The listing builds one solid part. Answer for the finished solid, in the listing's coordinates (mm). Face numbers are marked on the shaded views. A direction names the side the tool comes from. Coordinates: 2 decimals unless noted, no trailing zeros. Order: outer loops, then holes, each group sorted by start corner. A loop starts at its lowest first (then second) coordinate and runs counter-clockwise, first axis right, second up. Notation, with made-up numbers: (-20, 73.5) -> (22, 73.5) arc R13 cw to (22, 79.5) -> close; hole circle Ø2 at (-32, 11). An arc over 180 degrees is marked (long way). Return JSON: item names as keys, results as strings.
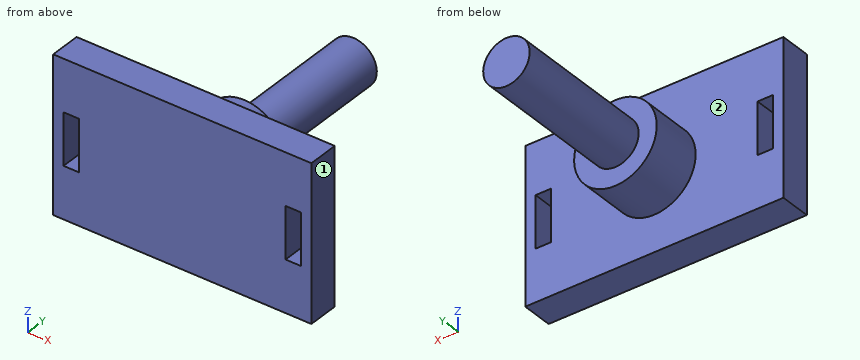
```python
from build123d import *

# Parameters (mm, degrees)
SKETCH1_R           = 2.25
BOSS_EXTRUDE1_DEPTH = 14
SKETCH2_R           = 4
BOSS_EXTRUDE2_DEPTH = 5
SKETCH3_W           = 25
SKETCH3_H           = 15
BOSS_EXTRUDE3_DEPTH = 3
SKETCH4_W           = 1.5
SKETCH4_H           = 5
CUT_EXTRUDE1_DEPTH  = 3


with BuildPart() as part:
    # Sketch1 → Boss-Extrude1 (new body)
    with BuildSketch(Plane(origin=(0, 0, 0), x_dir=(1, 0, 0), z_dir=(0, 1, 0))):
        with Locations(Location((0, 0, 0), (0, 0, 270))):
            Circle(SKETCH1_R)
    extrude(amount=BOSS_EXTRUDE1_DEPTH)

    # Sketch2 → Boss-Extrude2 (add)
    with BuildSketch(Plane.XZ):
        with Locations(Location((0, 0, 0), (0, 0, 270))):
            Circle(SKETCH2_R)
    extrude(amount=BOSS_EXTRUDE2_DEPTH)

    # Sketch3 → Boss-Extrude3 (add)
    with BuildSketch(Plane.XZ.offset(5)):
        Rectangle(SKETCH3_W, SKETCH3_H)
    extrude(amount=BOSS_EXTRUDE3_DEPTH)

    # Sketch4 → Cut-Extrude1 (cut)
    with BuildSketch(Plane.XZ.offset(8)):
        with Locations((-10.75, 0)):
            Rectangle(SKETCH4_W, SKETCH4_H)
        with Locations((10.75, 0)):
            Rectangle(SKETCH4_W, SKETCH4_H)
    extrude(amount=-CUT_EXTRUDE1_DEPTH, mode=Mode.SUBTRACT)


solid = part.part
```
Item 1: Find the intervals of material crossed by probe 1 along Z at (x, y) = (-11.25, -5.75); probe 2 along Y at (x, z) = (4.5, 5.5); probe 3 along X at (y, z) = (-1.5, -3.5), in increasing order.
Answer list:
{"probe 1": "-7.5 to -2.5, 2.5 to 7.5", "probe 2": "-8 to -5", "probe 3": "-1.94 to 1.94"}
Item 2: The part is cut by section D-D on y = -3.25. Determine the outline of the cut face in (x, z), plus the area to 3 significant figures.
Answer list:
{"outline": "circle Ø8 at (0, 0)", "area": "50.3 mm2"}
Item 3: The part is cut by section A-A on z = 0. Determine the outline of the cut face in (x, y), plus the area to 3 significant figures.
Answer list:
{"outline": "(-12.5, -8) -> (-11.5, -8) -> (-11.5, -5) -> (-12.5, -5) -> close; (-10, -8) -> (10, -8) -> (10, -5) -> (4, -5) -> (4, 0) -> (2.25, 0) -> (2.25, 14) -> (-2.25, 14) -> (-2.25, 0) -> (-4, 0) -> (-4, -5) -> (-10, -5) -> close; (11.5, -8) -> (12.5, -8) -> (12.5, -5) -> (11.5, -5) -> close", "area": "169 mm2"}
Item 4: The part is cut by section B-B on x = 0. Determine the outline of the cut face in (y, z), plus the area to 3 significant figures.
Answer list:
{"outline": "(-8, -7.5) -> (-5, -7.5) -> (-5, -4) -> (0, -4) -> (0, -2.25) -> (14, -2.25) -> (14, 2.25) -> (0, 2.25) -> (0, 4) -> (-5, 4) -> (-5, 7.5) -> (-8, 7.5) -> close", "area": "148 mm2"}
Item 5: The part is cut by section C-C on z = 5.5. Determine the outline of the cut face in (x, y).
Answer list:
{"outline": "(-12.5, -8) -> (12.5, -8) -> (12.5, -5) -> (-12.5, -5) -> close"}
Item 6: Which of the six approach directions +Z, -Z, +X, -X, +Y, -Y give full straight-line access (tool end or side, diameter ignored) to the marked faces 1 and 2?
Answer list:
{"face 1": "+Z, -Z, +X, +Y, -Y", "face 2": "+Y"}
Item 7: Flat-ended cylindrical pins translate along their axes: pin 1 (8 mm diameter, centred on x = 0.5, y = 3, fed in from -Z); pin 2 (4 mm diameter, centred on x = 2.5, y = 6.5, fed in from -Z). Find the tip coordinate at first contact, or state that the pin passes through.
Answer list:
{"pin 1": "z = -4", "pin 2": "z = -2.19"}
